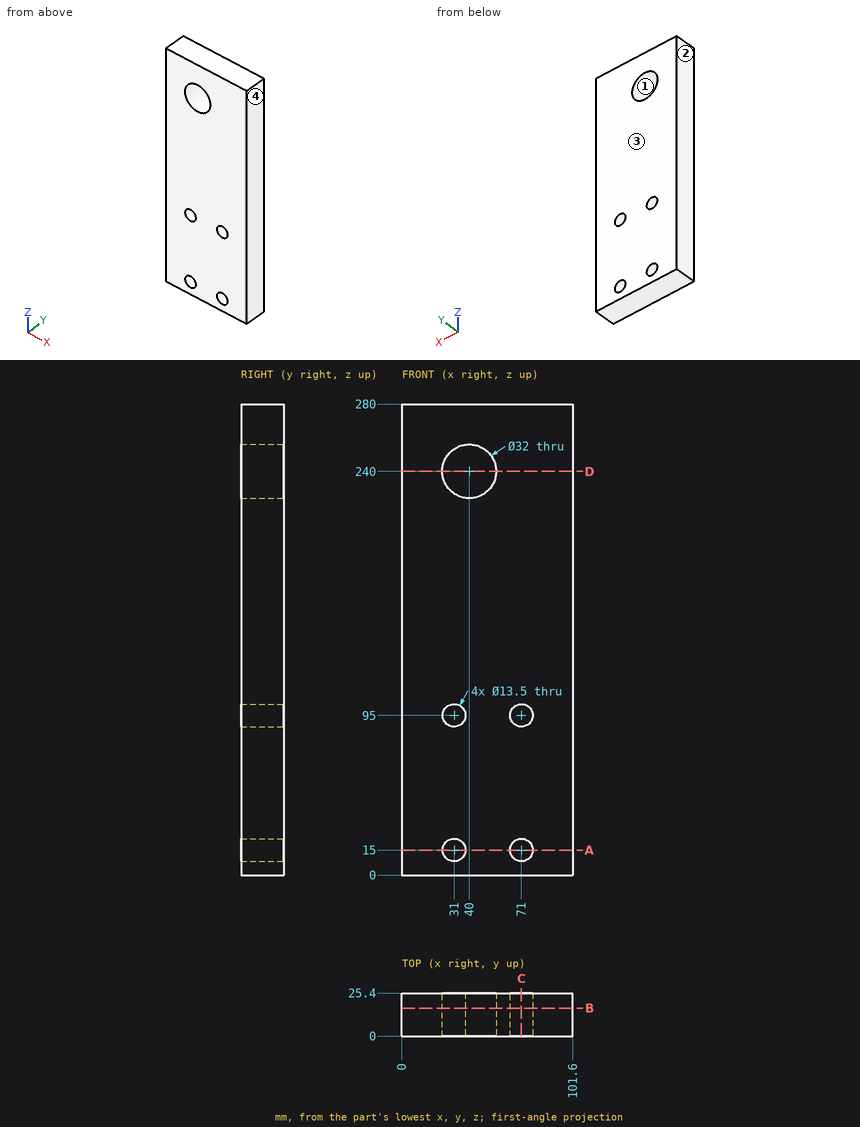
For this review, use the dimensioned drawing (mm, ordinates from the lowest corner) and the shaded views. Give positions to 0.01 mm unless a question says otherwise; leave off trailing zeros. Order: outer loops, then holes, each group sorted by start corner. A loop starts at its lowest first (then second) coordinate and runs counter-clockwise, first axis right, second up.
1. Add section D-D, the plane z = 240. State the section outline as (x, y) points.
Solution:
outline: (0, 0) - (24, 0) - (24, 25.4) - (0, 25.4) - close; (56, 0) - (101.6, 0) - (101.6, 25.4) - (56, 25.4) - close
2. Add section C-C, the plane x = 71. State the section outline as (y, z) points, then the cut area to 3 significant figures.
Solution:
outline: (0, 0) - (25.4, 0) - (25.4, 8.25) - (0, 8.25) - close; (0, 21.75) - (25.4, 21.75) - (25.4, 88.25) - (0, 88.25) - close; (0, 101.75) - (25.4, 101.75) - (25.4, 280) - (0, 280) - close
area: 6,430 mm2
3. Add section B-B, the plane y = 16.5. State the section outline as (x, z) points.
Solution:
outline: (0, 0) - (101.6, 0) - (101.6, 280) - (0, 280) - close; hole circle Ø32 at (40, 240); hole circle Ø13.5 at (31, 15); hole circle Ø13.5 at (31, 95); hole circle Ø13.5 at (71, 15); hole circle Ø13.5 at (71, 95)
4. For pin 1 Ø4 at (x, z) = (25.5, 36) entering from -Y; pin 2 Ø12 at (x, z) = (71, 15) entering from -Y, all flat-tipped, find the tip position at first contact; note any pin that passes through.
Solution:
pin 1: stops at y = 0
pin 2: passes through
5. Mouldability with a two-part tool opening along X and no side actions: class the marked faces 1, 2, 3 and 4 as +X half, -X half, draft (parallel to the pull), parting line (faces both ways), or undercut.
Solution:
face 1: undercut
face 2: -X half
face 3: draft
face 4: +X half
6. To check wall thickness, follow L1, parallel to X at y = 8.5, z = 15; L2, parallel to Z at x = 71, y = 5.75; L3, parallel to X at y = 12.25, z = 240. State the ranges of each line that lie inside material, in increasing order.
Solution:
L1: x = 0 to 24.25, 37.75 to 64.25, 77.75 to 101.6
L2: z = 0 to 8.25, 21.75 to 88.25, 101.75 to 280
L3: x = 0 to 24, 56 to 101.6
7. Add section A-A, the plane z = 15. State the section outline as (x, y) points, then the cut area to 3 significant figures.
Solution:
outline: (0, 0) - (24.25, 0) - (24.25, 25.4) - (0, 25.4) - close; (37.75, 0) - (64.25, 0) - (64.25, 25.4) - (37.75, 25.4) - close; (77.75, 0) - (101.6, 0) - (101.6, 25.4) - (77.75, 25.4) - close
area: 1,890 mm2
